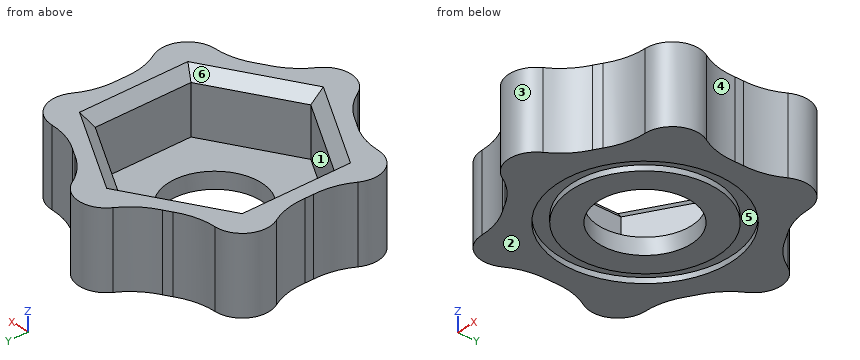
Autodesk Fusion 360 part; units mm, degrees
sketch "Sketch1" plane through (0, 0, 0) normal (0, 0, 1) x (1, 0, 0)
  circle A0 centre (0, 0) radius 8.5
  circle A1 centre (0, 0) radius 20
  dimension "d1" = 17
  dimension "d2" = 40
extrude "Extrude1" add sketch "Sketch1" along normal blind 14
sketch "Sketch2" plane through (0, 0, 14) normal (0, 0, 1) x (-1, 0, 0)
  circle A0 centre (0, 0) radius 8.5
  circle A1 centre (0, 0) radius 20
  line L0 (-15.25, -8.8046) -> (0, -17.6092)
  line L1 (0, -17.6092) -> (15.25, -8.8046)
  line L2 (15.25, -8.8046) -> (15.25, 8.8046)
  line L3 (15.25, 8.8046) -> (0, 17.6092)
  line L4 (0, 17.6092) -> (-15.25, 8.8046)
  line L5 (-15.25, 8.8046) -> (-15.25, -8.8046)
  line L6 (0, 0) -> (0, -24.7489) construction
  dimension "d5" = 15.25
extrude "Extrude2" cut sketch "Sketch2" against normal blind 11 contours L0 L1 L2 L3 L4 L5
sketch "Sketch3" plane through (0, 0, 14) normal (0, 0, 1) x (-1, 0, 0)
  line L0 (0, -17.6092) -> (-15.25, -8.8046)
  line L1 (-15.25, -8.8046) -> (-15.25, 8.8046)
  line L2 (-15.25, 8.8046) -> (0, 17.6092)
  line L3 (0, 17.6092) -> (15.25, 8.8046)
  line L4 (15.25, 8.8046) -> (15.25, -8.8046)
  line L5 (15.25, -8.8046) -> (0, -17.6092)
  circle A0 centre (0, 0) radius 20
  line L6 (0, -20) -> (0, 20) construction
  line L7 (20, 0) -> (-20, 0) construction
  arc A1 (-4.3301, -22.5) -> (4.3301, -22.5) centre (0, -20) ccw
  line L8 (0, -20) -> (0, -25) construction
  line L9 (0, -20) -> (4.3301, -22.5) construction
  line L10 (0, -20) -> (-4.3301, -22.5) construction
  arc A2 (9.3264, -17.6923) -> (4.3301, -22.5) centre (15.1554, -28.75) ccw
  arc A3 (-4.3301, -22.5) -> (-9.3264, -17.6923) centre (-15.1554, -28.75) ccw
  arc A4 (-9.3264, -17.6923) -> (9.3264, -17.6923) centre (0, 0) ccw
  arc A5 (17.3205, -15) -> (21.6506, -7.5) centre (17.3205, -10) ccw
  arc A6 (17.3205, -15) -> (10.6588, -16.9231) centre (17.3205, -27.5) ccw
  arc A7 (10.6588, -16.9231) -> (19.9852, -0.7692) centre (0, 0) ccw
  arc A8 (19.9852, -0.7692) -> (21.6506, -7.5) centre (32.476, -1.25) ccw
  arc A9 (21.6506, 7.5) -> (17.3205, 15) centre (17.3205, 10) ccw
  arc A10 (21.6506, 7.5) -> (19.9852, 0.7692) centre (32.476, 1.25) ccw
  arc A11 (19.9852, 0.7692) -> (10.6588, 16.9231) centre (0, 0) ccw
  arc A12 (10.6588, 16.9231) -> (17.3205, 15) centre (17.3205, 27.5) ccw
  arc A13 (4.3301, 22.5) -> (-4.3301, 22.5) centre (0, 20) ccw
  arc A14 (4.3301, 22.5) -> (9.3264, 17.6923) centre (15.1554, 28.75) ccw
  arc A15 (9.3264, 17.6923) -> (-9.3264, 17.6923) centre (0, 0) ccw
  arc A16 (-9.3264, 17.6923) -> (-4.3301, 22.5) centre (-15.1554, 28.75) ccw
  arc A17 (-17.3205, 15) -> (-21.6506, 7.5) centre (-17.3205, 10) ccw
  arc A18 (-17.3205, 15) -> (-10.6588, 16.9231) centre (-17.3205, 27.5) ccw
  arc A19 (-10.6588, 16.9231) -> (-19.9852, 0.7692) centre (0, 0) ccw
  arc A20 (-19.9852, 0.7692) -> (-21.6506, 7.5) centre (-32.476, 1.25) ccw
  arc A21 (-21.6506, -7.5) -> (-17.3205, -15) centre (-17.3205, -10) ccw
  arc A22 (-21.6506, -7.5) -> (-19.9852, -0.7692) centre (-32.476, -1.25) ccw
  arc A23 (-19.9852, -0.7692) -> (-10.6588, -16.9231) centre (0, 0) ccw
  arc A24 (-10.6588, -16.9231) -> (-17.3205, -15) centre (-17.3205, -27.5) ccw
  dimension "d10" = 60
  dimension "d11" = 60
  dimension "d12" = 5
  dimension "d14" = 360
extrude "Extrude3" add sketch "Sketch3" against normal up to surface (14 mm away) contours A0 A9 A10 A11 A12 | A0 A5 A6 A7 A8 | A0 A13 A14 A15 A16 | A0 A1 A2 A3 A4 | A0 A17 A18 A19 A20 | A0 A21 A22 A23 A24
chamfer "Chamfer1" distance 2 angle 45 6 edges at (-7.625, 13.2069, 14) (-15.25, 0, 14) (-7.625, -13.2069, 14) (7.625, -13.2069, 14) (15.25, 0, 14) (7.625, 13.2069, 14)
sketch "Sketch4" plane through (0, 0, 0) normal (0, 0, -1) x (1, 0, 0)
  circle A0 centre (0, 0) radius 8.5
  arc A1 (-9.3264, 17.6923) -> (-10.6588, 16.9231) centre (0, 0) ccw
  arc A2 (-17.3205, 15) -> (-10.6588, 16.9231) centre (-17.3205, 27.5) ccw
  arc A3 (-17.3205, 15) -> (-21.6506, 7.5) centre (-17.3205, 10) ccw
  arc A4 (-19.9852, 0.7692) -> (-21.6506, 7.5) centre (-32.476, 1.25) ccw
  arc A5 (-19.9852, 0.7692) -> (-19.9852, -0.7692) centre (0, 0) ccw
  arc A6 (-21.6506, -7.5) -> (-19.9852, -0.7692) centre (-32.476, -1.25) ccw
  arc A7 (-21.6506, -7.5) -> (-17.3205, -15) centre (-17.3205, -10) ccw
  arc A8 (-10.6588, -16.9231) -> (-17.3205, -15) centre (-17.3205, -27.5) ccw
  arc A9 (-10.6588, -16.9231) -> (-9.3264, -17.6923) centre (0, 0) ccw
  arc A10 (-4.3301, -22.5) -> (-9.3264, -17.6923) centre (-15.1554, -28.75) ccw
  arc A11 (-4.3301, -22.5) -> (4.3301, -22.5) centre (0, -20) ccw
  arc A12 (9.3264, -17.6923) -> (4.3301, -22.5) centre (15.1554, -28.75) ccw
  arc A13 (9.3264, -17.6923) -> (10.6588, -16.9231) centre (0, 0) ccw
  arc A14 (17.3205, -15) -> (10.6588, -16.9231) centre (17.3205, -27.5) ccw
  arc A15 (17.3205, -15) -> (21.6506, -7.5) centre (17.3205, -10) ccw
  arc A16 (19.9852, -0.7692) -> (21.6506, -7.5) centre (32.476, -1.25) ccw
  arc A17 (19.9852, -0.7692) -> (19.9852, 0.7692) centre (0, 0) ccw
  arc A18 (21.6506, 7.5) -> (19.9852, 0.7692) centre (32.476, 1.25) ccw
  arc A19 (21.6506, 7.5) -> (17.3205, 15) centre (17.3205, 10) ccw
  arc A20 (10.6588, 16.9231) -> (17.3205, 15) centre (17.3205, 27.5) ccw
  arc A21 (10.6588, 16.9231) -> (9.3264, 17.6923) centre (0, 0) ccw
  arc A22 (4.3301, 22.5) -> (9.3264, 17.6923) centre (15.1554, 28.75) ccw
  arc A23 (4.3301, 22.5) -> (-4.3301, 22.5) centre (0, 20) ccw
  arc A24 (-9.3264, 17.6923) -> (-4.3301, 22.5) centre (-15.1554, 28.75) ccw
  circle A25 centre (0, 0) radius 13.25
  circle A26 centre (0, 0) radius 15.75
  dimension "d18" = 26.5
  dimension "d19" = 31.5
extrude "Extrude4" cut sketch "Sketch4" against normal blind 1 contours A26
equation "d11 = d10"
Can you work these out from the model? Positions are in its coordinate system, mm. Face numbers are marked on the shaded views. A direction names the side the tool comes from. Round coordinates to 2 decimals unless told otherwise and drop trailing zeros. Loops run counter-clockwise (first coordinate to the right, second up) from the corner with the lowest first, then second, coordinate; pieces in that order, holes last. Notation, with made-up numbers: M 54.25,47 L 96.25,47 A22 cw 96.25,78 Z; hole C 86,84 d6. An arc over 180 degrees is marked long. Answer as a JSON object with one key per item and string values. Group by question number.
Q1. We'd pull the mould along Y, two halves only. Please class the marked faces 1, 2 and 3: +Y half, -Y half, draft (parallel to the pull), parting line (faces both ways), or undercut.
Q2. Will these pins go through, and if not, where does the flat tip stop? pin 1 (2.5 mm diameter, centred on y = 3, z = 9.5, fed in from -X); pin 2 (8 mm diameter, centred on x = 2.5, y = -8.5, fed in from +Z); pin 3 (8 mm diameter, centred on y = 2, z = 7.5, fed in from -X).
Q3. Please list where these lines run through material, in increasing order: L1, parallel to X at y = -17.5, z = 7.5; L2, parallel to Y at x = -1.5, z = 9; L3, parallel to X at y = -13, z = 5.5.
Q4. Imagine slicing it at D-D, the plane y = 14. Please give me the cut outline in (x, z).
Q5. On a 3-axis mill with a long thin cutter (end or side, diameter ignored), from which of +Z, -Z, +X, -X, +Y, -Y can I reach the whole of each face in a straight line? I mean the marked faces 4, 5 and 6. Say none if no direction works.
Q6. Imagine slicing it at A-A, the plane y = 0. Please give me the cut outline in (x, z), then the cut area to 4 significant figures.
Q7. Imagine slicing it at B-B, the plane x = 6. Please give me the cut outline in (y, z), then the cut area to 3 significant figures.
Findings:
{
 "1": {"face 1": "undercut", "face 2": "draft", "face 3": "-Y half"},
 "2": {"pin 1": "stops at x = -20.34", "pin 2": "stops at z = 3", "pin 3": "stops at x = -20.91"},
 "3": {"L1": "x = -9.68 to -0.19, 0.19 to 9.68", "L2": "y = -24.77 to -16.74, 16.74 to 24.77", "L3": "x = -21.32 to -7.98, 7.98 to 21.32"},
 "4": {"outline": "M -20.32,0 L -7.22,0 L -7.22,1 L 7.22,1 L 7.22,0 L 20.32,0 L 20.32,14 L 10.25,14 L 6.25,12 L 6.25,3 L -6.25,3 L -6.25,12 L -10.25,14 L -20.32,14 Z"},
 "5": {"face 4": "+Z, -Z, +X", "face 5": "-Z", "face 6": "+Z"},
 "6": {"outline": "M -20,0 L -15.75,0 L -15.75,1 L -13.25,1 L -13.25,0 L -8.5,0 L -8.5,3 L -15.25,3 L -15.25,12 L -17.25,14 L -20,14 Z; M 8.5,0 L 13.25,0 L 13.25,1 L 15.75,1 L 15.75,0 L 20,0 L 20,14 L 17.25,14 L 15.25,12 L 15.25,3 L 8.5,3 Z", "area": "164.5 mm2"},
 "7": {"outline": "M -20.24,0 L -14.56,0 L -14.56,1 L -11.81,1 L -11.81,0 L -6.02,0 L -6.02,3 L -14.15,3 L -14.15,12 L -16.45,14 L -20.24,14 Z; M 6.02,0 L 11.81,0 L 11.81,1 L 14.56,1 L 14.56,0 L 20.24,0 L 20.24,14 L 16.45,14 L 14.15,12 L 14.15,3 L 6.02,3 Z", "area": "209 mm2"}
}
